from build123d import *

# Parameters (mm, degrees)
EXTRUDE_THIN1_DEPTH            = 25.4
F_9_0_196_DIAMETER_HOLE1_D     = 4.9784
F_9_0_196_DIAMETER_HOLE1_DEPTH = 1.5885


with BuildPart() as part:
    # Sketch1 → Extrude-Thin1 (new body)
    with BuildSketch(Plane.XY):
        Polygon((0, -25.4), (0, 0), (15.981992956, 19.741729943), (17.215851078, 18.742855383), (1.5875, -0.562039024), (1.5875, -25.4), align=None)
    extrude(amount=-EXTRUDE_THIN1_DEPTH)

    # #9 (0.196) Diameter Hole1
    with Locations(Plane(origin=(1.233858121, -0.99887456, 0), x_dir=(0, 0, -1), z_dir=(0.777233462, -0.629212321, 0))):
        with Locations((12.7, 12.7)):
            f_9_0_196_diameter_hole1 = Hole(F_9_0_196_DIAMETER_HOLE1_D / 2, depth=F_9_0_196_DIAMETER_HOLE1_DEPTH)

    # Mirror1: #9 (0.196) Diameter Hole1 across plane
    add(f_9_0_196_diameter_hole1.mirror(Plane(origin=(0, 0, 0), x_dir=(0, 0, 1), z_dir=(-0.33374132, -0.942664697, 0))), mode=Mode.SUBTRACT)


solid = part.part
Verification items for the finished model (mm, model axes). A direction names the side the tool comes from. Give positions to 0.01 mm unless a question says otherwise; leave off trailing zeros. Loops run counter-clockwise (first coordinate to the right, second up) from the corner with the lowest first, then second, coordinate; pieces in that order, holes last. Notation, with made-up numbers: (-35, 17) - (-30, 17) arc R27 cw to (-30, 35) - close; hole circle Ø9 at (66.25, -7.5). An arc over 180 degrees is marked (long way). Write each question's results on one line, items separated by ' | '.
1) Sectioned sample at A-A on y = -12.7. Record the boundary of the cut face in (x, z), plus the area to 3 significant figures.
Solution:
outline: (0, -25.4) - (1.59, -25.4) - (1.59, -15.19) - (0, -15.19) - close; (0, -10.21) - (1.59, -10.21) - (1.59, 0) - (0, 0) - close | area: 32.4 mm2
2) Sectioned sample at D-D on y = 5.5. Record the boundary of the cut face in (x, z).
Solution:
outline: (4.45, -25.4) - (6.5, -25.4) - (6.5, 0) - (4.45, 0) - close
3) Tool access check on faces 1 (the flat face through (1, -25.4, -13)), 2 (the flat face through (1.588, -10, -13)). Record the directions out of +Z, -Z, +X, -X, +Y, -Y that give a thin tool (end or side, any length) a straight path to the whole face; none if there is none.
Solution:
face 1: +Z, -Z, +X, -X, -Y | face 2: +Z, -Z, +X, -Y
4) Sectioned sample at B-B on z = -12.7. Record the boundary of the cut face in (x, y).
Solution:
outline: (0, -25.4) - (1.59, -25.4) - (1.59, -15.19) - (0, -15.19) - close; (0, -10.21) - (1.59, -10.21) - (1.59, -0.56) - (7.66, 6.94) - (6.42, 7.94) - (0, 0) - close; (9.56, 11.81) - (10.79, 10.81) - (17.22, 18.74) - (15.98, 19.74) - close
5) Material ranges on L1, parallel to X at y = -7.5, z = -10.75; L2, parallel to Y at x = 0.55, z = -12.7; L3, parallel to Y at x = 0.5, z = -12.7, recorded low to high. Write a range as from..to.
Solution:
L1: 0..1.59 | L2: -25.4..-15.19, -10.21..0.68 | L3: -25.4..-15.19, -10.21..0.62
6) Mould release check, pull along Z, two halves, no side actions. Record for faces 3 (the cylindrical face through (9.92, 11.01, -11.36)), 4 (the flat face through (2, 1, 0)), 5 (the flat face through (16.59, 19.25, -12.52)): pulls with the +Z half, pulls with the -Z half, needs draft (parallel to the pull), parting line crosses it, or undercut.
Solution:
face 3: undercut | face 4: pulls with the +Z half | face 5: needs draft
7) Depth check by flat-ended pin: P1, Ø5, axis at x = 8.5, z = -4, coming from the -Y side; P2, Ø6, axis at x = 15, z = -12, coming from the -Y side; P3, Ø7.5, axis at y = -16, z = -9.5, coming from the +X side. Enter the tip coordinate at first touch or a pass-through.
Solution:
P1: y = 4.89 | P2: y = 12.3 | P3: x = 1.59
8) Sectioned sample at C-C on z = -2. Record the boundary of the cut face in (x, y), plus the area to 3 significant figures.
Solution:
outline: (0, -25.4) - (1.59, -25.4) - (1.59, -0.56) - (17.22, 18.74) - (15.98, 19.74) - (0, 0) - close | area: 79.8 mm2
